Autodesk Inventor part; units mm, degrees
ref_plane "YZ Plane" through (0, 0, 0) normal (1, 0, 0) x (0, 1, 0)
ref_plane "XZ Plane" through (0, 0, 0) normal (0, 1, 0) x (-1, 0, 0)
ref_plane "XY Plane" through (0, 0, 0) normal (0, 0, 1) x (1, 0, 0)
sketch "Sketch1" plane through (0, 0, 0) normal (1, 0, 0) x (0, 1, 0)
  line L0 (0, 0) -> (40, -0.6982)
  line L1 (40, -0.6982) -> (39.9486, -3.6454)
  line L2 (39.9486, -3.6454) -> (36.9486, -3.6454)
  line L3 (36.9486, -3.6454) -> (2, -3.0354)
  line L4 (2, -3.0354) -> (2, -16.7514)
  line L5 (2, -16.7514) -> (40, -16.7514)
  line L6 (40, -16.7514) -> (40, -19.7514)
  line L7 (40, -19.7514) -> (0, -19.7514)
  line L8 (0, -19.7514) -> (0, 0)
  line L9 (10, -16.7514) -> (10, -15.7514)
  line L10 (10, -15.7514) -> (2, -15.7514)
  line L11 (39.9486, -3.6454) -> (39.4486, -4.5114)
  line L12 (39.9486, -3.6454) -> (40.9486, -3.6454) construction
  line L13 (39.4486, -4.5114) -> (38.9486, -3.6454)
  line L14 (36.9486, -3.6454) -> (37.4486, -4.5114)
  line L15 (37.4486, -4.5114) -> (37.9486, -3.6454)
  line L16 (37.9486, -3.6454) -> (38.4486, -4.5114)
  line L17 (38.4486, -4.5114) -> (38.9486, -3.6454)
  line L18 (0, -5.2681) -> (1, -5.2681)
  line L19 (1, -5.2681) -> (1, -14.2681)
  line L20 (1, -14.2681) -> (0, -14.2681)
  dimension "d5" = 40
  dimension "d6" = 13.716
  dimension "d7" = 3
  dimension "d8" = 3
  dimension "d9" = 40
  dimension "d10" = 3
  dimension "d11" = 2
  dimension "d12" = 89
  dimension "d13" = 1
  dimension "d14" = 30
  dimension "d15" = 1
  dimension "d16" = 120
  dimension "d17" = 120
  dimension "d18" = 60
  dimension "d19" = 60
  dimension "d20" = 1
  dimension "d33" = 1
  dimension "d34" = 9
extrude "Extrusion1" add sketch "Sketch1" along normal blind 25
sketch "Sketch2" plane through (0, 0, -19.7514) normal (0, 0, -1) x (-1, 0, 0)
  line L0 (0, 10) -> (-25, 10)
  line L1 (-25, 10) -> (0, 0)
  line L2 (-7.459, 5) -> (-9.9795, 0.6344)
  line L3 (-9.9795, 0.6344) -> (-15.0205, 0.6344)
  line L4 (-15.0205, 0.6344) -> (-17.541, 5)
  line L5 (-17.541, 5) -> (-15.0205, 9.3656)
  line L6 (-15.0205, 9.3656) -> (-9.9795, 9.3656)
  line L7 (-9.9795, 9.3656) -> (-7.459, 5)
  point P0 (-12.5, 5)
  dimension "d23" = 8.7312
extrude "Extrusion2" cut sketch "Sketch2" against normal blind 3.175
sketch "Sketch3" plane through (0, 0, -16.5764) normal (0, 0, -1) x (-1, 0, 0)
  point P0 (0, 0)
  point P1 (-12.5, 5)
hole "Hole1" at (12.5, 5, -16.5764) direction (0, 0, 1) diameter 4.4958 end through all
sketch "Sketch4" plane through (0, 0, 0) normal (-1, 0, 0) x (0, 0, 1)
  line L0 (-19.7514, 0) -> (-19.7514, 40)
  line L1 (0, 0) -> (-19.7514, 0)
  line L2 (-7.2514, 0) -> (-16.2514, 0)
  line L3 (-16.2514, 0) -> (-16.2514, 1)
  line L4 (-16.2514, 1) -> (-7.2514, 1)
  line L5 (-7.2514, 1) -> (-7.2514, 0)
  dimension "d35" = 9
  dimension "d36" = 1
  dimension "d38" = 3.5
extrude "Extrusion3" cut sketch "Sketch4" against normal through all
equation "\"d6\" = StretcherDepth"
equation "\"d8\" = d7"
equation "\"d9\" = d5"
properties part number "MotorClip"
Design review of the part built by this model. Coordinates are the model's own, in mm. A direction names the side the tool comes from. Coordinates: 2 decimals unless noted, no trailing zeros. Loops run counter-clockwise (first coordinate to the right, second up) from the corner with the lowest first, then second, coordinate; pieces in that order, holes last. Notation, with made-up numbers: (-30, 1) - (20, 1) arc R20 ccw to (20, 37) - close; hole circle Ø1 at (62, 70.25). An arc over 180 degrees is marked (long way). Use CSV: the item, a comma, the result in double quotes. Start each with the question number.
1. Add section B-B on x = 1.75. Give the boundary of the cut face in (y, z).
2. Mouldability with a two-part tool opening along X and no side actions: class faces 4 (the flat face through (11, 7, -16.576)), 5 (the flat face through (12.3, 0.5, -7.251)), 6 (the flat face through (25, 15, -3)) as released by +X, released by -X, zero draft, split by the parting line, or undercut.
3. Add section A-A on y = 21. Give the boundary of the cut face in (x, z).
4. To check wall thickness, follow probe 1 along X at (y, z) = (5, -2.25); probe 2 along Y at (x, z) = (12.5, -0.8); probe 3 along Y at (x, z) = (12.5, -16.35). State the ranges of each line that lie inside material, in increasing order.
5. Add section D-D on x = 12.5. Count the separate pieces of the cut face and the enclosed holes in it, plus the area to 3 significant figures.
6. For faces 1 (the flat face through (12, 1, -12)), 2 (the flat face through (12.325, 37.195, -4.072)), 3 (the flat face through (13, 9.366, -18)), list the 3-axis set-ups (+Z, -Z, +X, -X, +Y, -Y) from which the entire face can be reached by the end or side of a thin tool; tool diameter is ignored.
7. Add section C-C on y = 6.5. Give the boundary of the cut face in (x, z).
8. Clearance check with flat-ended pins moving along their axes: pin 1 (7.5 mm diameter, centred on x = 6.5, y = 18, fed in from +Z); pin 2 (7 mm diameter, centred on x = 12.5, y = 5, fed in from +Z); pin 3 (1.5 mm diameter, centred on x = 3, z = -15, fed in from -Y). State where each tip first meets the part, or that it passes through.
Resolved:
1,outline,"(0, -19.75) - (40, -19.75) - (40, -16.75) - (10, -16.75) - (10, -15.75) - (2, -15.75) - (2, -3.04) - (36.95, -3.65) - (37.45, -4.51) - (37.95, -3.65) - (38.45, -4.51) - (38.95, -3.65) - (39.45, -4.51) - (39.95, -3.65) - (40, -0.7) - (0, 0) - (0, -7.25) - (1, -7.25) - (1, -16.25) - (0, -16.25) - close"
2,face 4,"undercut"
2,face 5,"zero draft"
2,face 6,"released by +X"
3,outline,"(0, -19.75) - (25, -19.75) - (25, -16.75) - (0, -16.75) - close; (0, -3.37) - (25, -3.37) - (25, -0.37) - (0, -0.37) - close"
4,probe 1,"0 to 10.25, 14.75 to 25"
4,probe 2,"0 to 2.75, 7.25 to 40"
4,probe 3,"0 to 2.75, 7.25 to 10"
5,separate pieces,"3"
5,enclosed holes,"0"
5,area,"223 mm2"
6,face 1,"+X, -X, -Y"
6,face 2,"+X, -X"
6,face 3,"-Z"
7,outline,"(0, -19.75) - (8.33, -19.75) - (8.33, -16.58) - (10.83, -16.58) - (10.83, -15.75) - (0, -15.75) - close; (0, -3.11) - (10.83, -3.11) - (10.83, -0.11) - (0, -0.11) - close; (14.17, -16.58) - (16.67, -16.58) - (16.67, -19.75) - (25, -19.75) - (25, -15.75) - (14.17, -15.75) - close; (14.17, -3.11) - (25, -3.11) - (25, -0.11) - (14.17, -0.11) - close"
8,pin 1,"z = -0.25"
8,pin 2,"z = -0.03"
8,pin 3,"y = 1"
